from build123d import *

# Parameters (mm, degrees)
SKETCH1_R           = 0.5
SKETCH1_R_2         = 0.501124618
BOSS_EXTRUDE1_DEPTH = 2


with BuildPart() as part:
    # Sketch1 → Boss-Extrude1 (new body)
    with BuildSketch(Plane(origin=(3.665299607, -3164.606366481, 1.228377955), x_dir=(1, 0, 0), z_dir=(0, 1, 0))):
        with BuildLine():
            Line((28.210288662, -32.620192101), (30.210288662, -32.620192101))
            Line((30.210288662, -32.620192101), (30.210288662, -8.620192101))
            Line((30.210288662, -8.620192101), (28.210288662, -8.620192101))
            Line((28.210288662, -8.620192101), (-3.789711338, -8.620192101))
            ThreePointArc((-3.789711338, -8.620192101), (-14.744162488, -11.88699157), (-22.120014118, -20.620192101))
            ThreePointArc((-22.120014118, -20.620192101), (-14.744162488, -29.353392632), (-3.789711338, -32.620192101))
            Line((-3.789711338, -32.620192101), (28.210288662, -32.620192101))
        make_face()
        with Locations((-19.129616691, -20.617828064)):
            Circle(SKETCH1_R, mode=Mode.SUBTRACT)
        with Locations((24.75459638, -20.617828064)):
            Circle(SKETCH1_R, mode=Mode.SUBTRACT)
        with Locations((10.8879759, -20.617828064)):
            Circle(SKETCH1_R_2, mode=Mode.SUBTRACT)
        with Locations((-3.377772721, -20.597275642)):
            Circle(SKETCH1_R, mode=Mode.SUBTRACT)
    extrude(amount=BOSS_EXTRUDE1_DEPTH)


solid = part.part
Could you check a few things on this model? Use its own coordinates, in mm. Give positions to 0.01 mm unless a question says otherwise; leave off trailing zeros. Loops run counter-clockwise (first coordinate to the right, second up) from the corner with the lowest first, then second, coordinate; pieces in that order, holes last. Notation, with made-up numbers: M -6,-13.5 L 35,-13.5 A19 ccw 35,23.5 Z; hole C 36.5,-38.75 d2. An arc over 180 degrees is marked long. Answer as a JSON object with one key per item and string values.
Q1. If I drill on probe 1 along Z at (x, y) = (-12.5, -3162.85); probe 2 along Z at (x, y) = (-11.5, -3163.7); probe 3 along X at (y, z) = (-3162.9, 27.5), over which ranges is the centre line in solid material (lowest first)? Write a range as [from, to].
Values found:
{"probe 1": "z = [14.14, 29.56]", "probe 2": "z = [13.4, 30.3]", "probe 3": "x = [-14.74, 33.88]"}
Q2. If we mould it in two halves opening along X, with no side actions, what happens to faces 1 (the flat face through (7, -3164.606, 22)), 2 (the cylindrical face through (-15.23, -3163.62, 22.29)), 3 (the flat face through (33.876, -3164, 22))? For each: pulls with the +X half, pulls with the -X half, needs draft (parallel to the pull), parting line crosses it, or undercut.
Values found:
{"face 1": "needs draft", "face 2": "undercut", "face 3": "pulls with the +X half"}
Q3. Suppose I cut it at A-A, the plane y = -3163.85. List the corners of the cut face in (x, z) for me, plus the area to 3 significant figures.
Values found:
{"outline": "M -18.45,21.85 A20 ccw -0.12,9.85 L 33.88,9.85 L 33.88,33.85 L -0.12,33.85 A20 ccw Z; hole C -15.46,21.85 d1; hole C 0.29,21.83 d1; hole C 14.55,21.85 d1; hole C 28.42,21.85 d1", "area": "1,130 mm²"}
Q4. Suppose I cut it at B-B, the plane z = 19.25. List the corners of the cut face in (x, y) for me.
Values found:
{"outline": "M -17.09,-3164.61 L 33.88,-3164.61 L 33.88,-3162.61 L -17.09,-3162.61 Z"}
Q5. Suppose I cut it at C-C, the plane z = 30. List the corners of the cut face in (x, y) for me.
Values found:
{"outline": "M -11.92,-3164.61 L 33.88,-3164.61 L 33.88,-3162.61 L -11.92,-3162.61 Z"}
Q6. For P1, Ø0.8, axis at x = 14.55, z = 21.85, coming from the +Y side, with a flat end and sliding along its axis, tell me the tip position at first contact or that it passes through.
Values found:
{"P1": "passes through"}
